Check sheet for the drawn part. Datum: minimum x, y, z corner. Units: mm. A direction names the side the tool comes from. Coordinates: 2 decimals unless noted, no trailing zeros. Write each loop counter-clockwise with the first axis right and the second up, starting at its lowest first coordinate (ties: lowest second). Pieces come first, ordered by that corner, then holes. Notation, with made-up numbers: M 34.25,48 L 58.25,48 A23 cw 58.25,81 Z; hole C -21,41.5 d6. An arc over 180 degrees is marked long. Answer as CSV lines item,"result". Start each with the question number.
Q1. Sectioned sample at C-C, the plane y = 8.75. Record the cut outline in (x, z), then the cut area to 3 significant figures.
Q2. Access from +Z, -Z, +X, -X, +Y, -Y to the whole of each face (thin tool, end or side, straight path). Record for the marked faces 1, 2, 3, 4 and 5.
Q3. Depth check by flat-ended pin: pin 1 Ø6 at (x, z) = (52.5, 42) entering from +Y; pin 2 Ø22 at (x, z) = (44.5, 34) entering from -Y; pin 3 Ø12 at (y, z) = (18, 33.5) entering from -X. Enter the tip coordinate at first touch or a pass-through.
Q4. Thickness scan on line 1 along Y through (x, z) = (41.5, 40.5); line 2 along Z through (x, y) = (12, 16.75); line 3 along X through (y, z) = (10.5, 42.5). Record the ranges inside material, lowest first. Write a range as from..to.
Q5. Sectioned sample at D-D, the plane z = 4. Record the cut outline in (x, y).
Q6. Sectioned sample at B-B, the plane z = 38. Record the cut outline in (x, y), then the cut area to 3 significant figures.
Q7. Sectioned sample at A-A, the plane x = 10. Record the cut outline in (y, z), then the cut area to 3 significant figures.
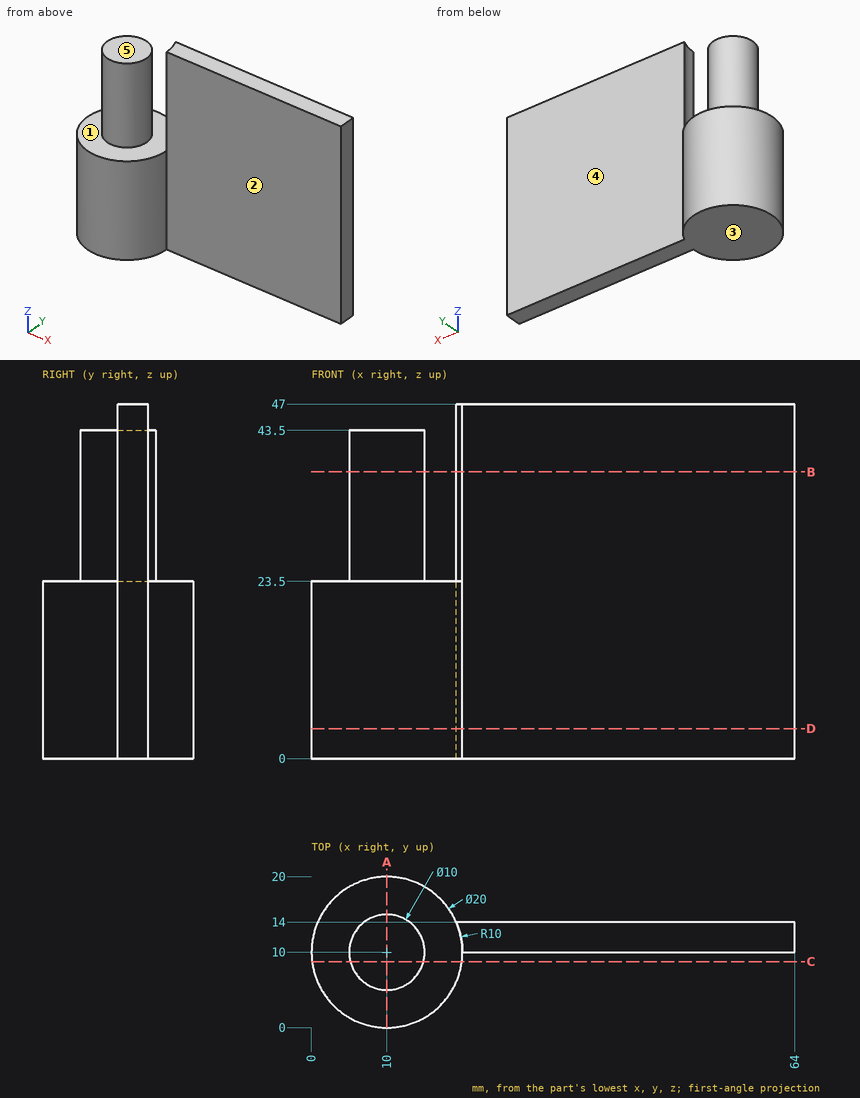
Output:
1,outline,"M 0.08,0 L 19.92,0 L 19.92,23.5 L 14.84,23.5 L 14.84,43.5 L 5.16,43.5 L 5.16,23.5 L 0.08,23.5 Z"
1,area,"660 mm^2"
2,face 1,"+Z"
2,face 2,"+Z, -Z, +X, -Y"
2,face 3,"-Z, +X, -X, +Y, -Y"
2,face 4,"+Z, -Z, +X, +Y"
2,face 5,"+Z, -X, +Y, -Y"
3,pin 1,"stops at y = 14"
3,pin 2,"stops at y = 10"
3,pin 3,"stops at x = 5.42"
4,line 1,"y = 10..14"
4,line 2,"z = 0..23.5"
4,line 3,"x = 5.03..14.97, 19.99..64"
5,outline,"M 19.17,14 A10 ccw long 20,10 L 64,10 L 64,14 Z"
6,outline,"C 10,10 d10; M 19.17,14 A10 cw 20,10 L 64,10 L 64,14 Z"
6,area,"256 mm^2"
7,outline,"M 0,0 L 20,0 L 20,23.5 L 15,23.5 L 15,43.5 L 5,43.5 L 5,23.5 L 0,23.5 Z"
7,area,"670 mm^2"
